Verification items for this drawing (mm, ordinates from the low corner). Round coordinates to 2 decimals unless told otherwise and drop trailing zeros. Write each loop counter-clockwise with the first axis right and the second up, starting at its lowest first coordinate (ties: lowest second). Pieces come first, ordered by that corner, then holes.
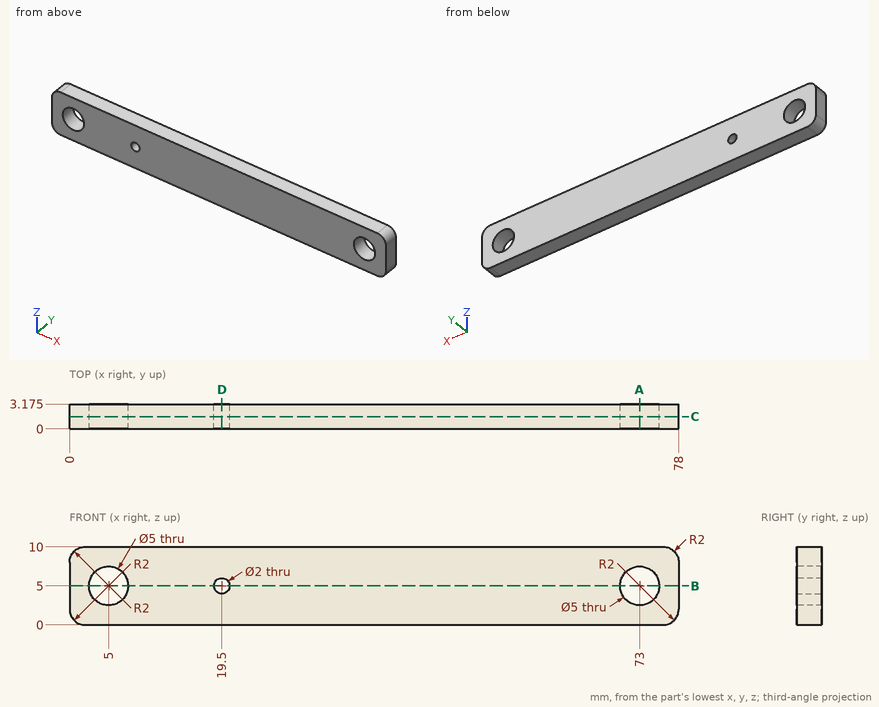
1. Section check A-A (x = 73). Record the cut outline in (y, z) (3 decimals).
2. Depth check by flat-ended pin: pin 1 Ø3 at (x, z) = (19, 5.5) entering from -Y; pin 2 Ø4.5 at (x, z) = (73, 5) entering from +Y. Enter the tip coordinate at first touch or a pass-through.
3. Section check D-D (x = 19.5). Record the cut outline in (y, z) (3 decimals), plus the area to 3 significant figures.
4. Section check C-C (y = 1.55). Record the cut outline in (x, z).
5. Scan lines: line 1 along X through (y, z) = (2.1, 5); line 2 along X through (y, z) = (0.2, 4.25); line 3 along X through (y, z) = (0.25, 1.75). Record each from-to range of solid material in increasing order.
6. Section check B-B (z = 5). Record the cut outline in (x, y) (3 decimals), plus the area to 3 significant figures.
Results below:
1. outline: (0, 0) - (3.175, 0) - (3.175, 2.5) - (0, 2.5) - close; (0, 7.5) - (3.175, 7.5) - (3.175, 10) - (0, 10) - close
2. pin 1: stops at y = 0
2. pin 2: passes through
3. outline: (0, 0) - (3.175, 0) - (3.175, 4) - (0, 4) - close; (0, 6) - (3.175, 6) - (3.175, 10) - (0, 10) - close
3. area: 25.4 mm2
4. outline: (0, 2) arc R2 ccw to (2, 0) - (76, 0) arc R2 ccw to (78, 2) - (78, 8) arc R2 ccw to (76, 10) - (2, 10) arc R2 ccw to (0, 8) - close; hole circle Ø5 at (5, 5); hole circle Ø2 at (19.5, 5); hole circle Ø5 at (73, 5)
5. line 1: x = 0 to 2.5, 7.5 to 18.5, 20.5 to 70.5, 75.5 to 78
5. line 2: x = 0 to 2.62, 7.38 to 18.84, 20.16 to 70.62, 75.38 to 78
5. line 3: x = 0.02 to 77.98
6. outline: (0, 0) - (2.5, 0) - (2.5, 3.175) - (0, 3.175) - close; (7.5, 0) - (18.5, 0) - (18.5, 3.175) - (7.5, 3.175) - close; (20.5, 0) - (70.5, 0) - (70.5, 3.175) - (20.5, 3.175) - close; (75.5, 0) - (78, 0) - (78, 3.175) - (75.5, 3.175) - close
6. area: 210 mm2
